from build123d import *

# Parameters (mm, degrees)
BOSS_EXTRUDE3_DEPTH = 15
SKETCH3_R           = 4
CUT_EXTRUDE3_DEPTH  = 14.0462
CUT_EXTRUDE4_DEPTH  = 3


with BuildPart() as part:
    # Sketch1 → Boss-Extrude3 (new body)
    with BuildSketch(Plane.YZ):
        with BuildLine():
            Line((-28.968617751, -12.789334175), (28.968617751, -12.789334175))
            ThreePointArc((28.968617751, -12.789334175), (44.579120821, 0), (35.110840206, 17.821518929))
            ThreePointArc((35.110840206, 17.821518929), (30.644623053, 21.505675602), (28.968617751, 27.047436358))
            Line((28.968617751, 27.047436358), (28.968617751, 39.053986921))
            ThreePointArc((28.968617751, 39.053986921), (26.039685563, 46.125054733), (18.968617751, 49.053986921))
            Line((18.968617751, 49.053986921), (-18.968617751, 49.053986921))
            ThreePointArc((-18.968617751, 49.053986921), (-26.039685563, 46.125054733), (-28.968617751, 39.053986921))
            Line((-28.968617751, 39.053986921), (-28.968617751, 27.047436358))
            ThreePointArc((-28.968617751, 27.047436358), (-30.644623053, 21.505675602), (-35.110840206, 17.821518929))
            ThreePointArc((-35.110840206, 17.821518929), (-44.579120821, 0), (-28.968617751, -12.789334175))
        make_face()
    extrude(amount=BOSS_EXTRUDE3_DEPTH)

    # Sketch3 → Cut-Extrude3 (cut)
    with BuildSketch(Plane.YZ.offset(15)):
        with Locations(Location((0, 3.132326373, 0), (0, 0, 270))):
            Circle(SKETCH3_R)
    extrude(amount=-CUT_EXTRUDE3_DEPTH, mode=Mode.SUBTRACT)

    # Sketch4 → Cut-Extrude4 (cut)
    with BuildSketch(Plane.YZ.offset(15)):
        with BuildLine():
            Line((-12.95, 49.053986921), (-12.95, 31.267703884))
            ThreePointArc((-12.95, 31.267703884), (0, 18.317703884), (12.95, 31.267703884))
            Line((12.95, 31.267703884), (12.95, 49.053986921))
            Line((12.95, 49.053986921), (-12.95, 49.053986921))
        make_face()
    extrude(amount=-CUT_EXTRUDE4_DEPTH, mode=Mode.SUBTRACT)


solid = part.part
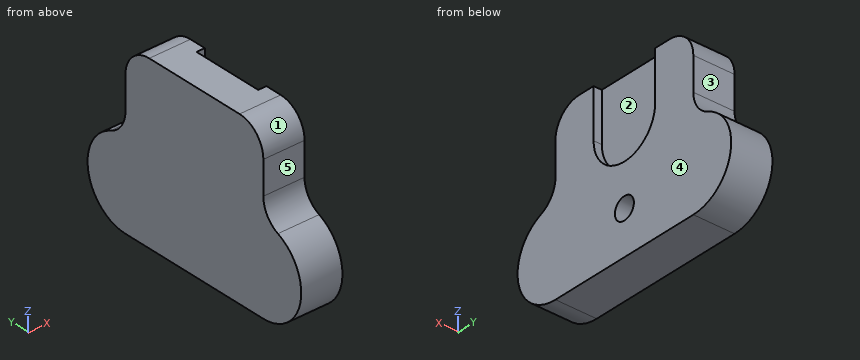
Geometry check sheet. Reference: the model listing, model coordinates, mm. Face numbers are marked on the shaded views. A direction names the side the tool comes from. Round coordinates to 2 decimals unless told otherwise and drop trailing zeros. Order: outer loops, then holes, each group sorted by start corner. A loop starts at its lowest first (then second) coordinate and runs counter-clockwise, first axis right, second up. Notation, with made-up numbers: M 63,3 L 91,3 A25 ccw 91,32 Z; hole C 52,79.25 d6. An arc over 180 degrees is marked long. Write each question's results on one line, items separated by ' | '. Start each with the question number.
1. Cross-section at D-D on y = -9. Record the boundary of the cut face in (x, z).
2. Cross-section at B-B on y = 0. Record the boundary of the cut face in (x, z).
3. Go/stop test with flat-tipped pins: P1, Ø3.5, axis at x = 13, z = 39.5, coming from the -Y side; P2, Ø13, axis at y = 5.5, z = 32.5, coming from the +X side; P3, Ø3.5, axis at x = 14, z = 43.5, coming from the +Y side. Record where each tip stops, or that it passes through.
4. Set-up check for the marked faces 4 and 5: record each of +Z, -Z, +X, -X, +Y, -Y from which the full face is reachable in a straight line by a thin tool's end or side.
5. Material ranges on L1, parallel to X at y = -11, z = 37.5; L2, parallel to Z at x = 13.75, y = 1.5; L3, parallel to Z at x = 5, y = 3.5, recorded low to high. Write a range as from..to.
6. Draft check along Y on the marked faces 1, 2 and 3. Enter one of: pulls with the +Y half, pulls with the -Y half, needs draft (parallel to the pull), parting line crosses it, or undercut.
7. Cross-section at C-C on z = 42.5. Record the boundary of the cut face in (x, y).
8. Cross-section at A-A on x = 7. Record the boundary of the cut face in (y, z), plus the area to 3 significant figures.
Resolved:
1) outline: M 0,-12.79 L 15,-12.79 L 15,21.96 L 12,21.96 L 12,49.05 L 0,49.05 Z
2) outline: M 0,-12.79 L 15,-12.79 L 15,-0.87 L 0.95,-0.87 L 0.95,7.13 L 15,7.13 L 15,18.32 L 12,18.32 L 12,49.05 L 0,49.05 Z
3) P1: y = -28.97 | P2: x = 12 | P3: y = 28.6
4) face 4: +Z, -Z, +X, +Y, -Y | face 5: +Z, +X, -X, -Y
5) L1: 0..12 | L2: -12.79..-0.58, 6.84..18.4 | L3: -12.79..1.2, 5.07..49.05
6) face 1: pulls with the -Y half | face 2: undercut | face 3: pulls with the +Y half
7) outline: M 0,-28.36 L 15,-28.36 L 15,-12.95 L 12,-12.95 L 12,12.95 L 15,12.95 L 15,28.36 L 0,28.36 Z
8) outline: M -35.11,17.82 A15.92 ccw -28.97,-12.79 L 28.97,-12.79 A15.92 ccw 35.11,17.82 A10 cw 28.97,27.05 L 28.97,39.05 A10 ccw 18.97,49.05 L -18.97,49.05 A10 ccw -28.97,39.05 L -28.97,27.05 A10 cw Z; hole C 0,3.13 d8 | area: 4,310 mm2
